Design review of the part built by this model. Coordinates are the model's own, in mm. A direction names the side the tool comes from. Give positions to 0.01 mm unless a question says otherwise; leave off trailing zeros. Order: outer loops, then holes, each group sorted by start corner. A loop starts at its lowest first (then second) coordinate and runs counter-clockwise, first axis right, second up. Notation, with made-up numbers: (22.5, 63) -> (36.5, 63) arc R29 ccw to (36.5, 99) -> close; hole circle Ø11 at (83.25, -6). An arc over 180 degrees is marked (long way). One line per item, written item: value.
from build123d import *

# Parameters (mm, degrees)
F0_R      = 3.175
F1_DEPTH  = 76.2
F2_R      = 3.175
F3_DEPTH  = 25.4
F3_FACE_R = 3.175
F4_DEPTH  = 50.8


with BuildPart() as f1:
    # F0 (on Front) → F1 (new body)
    with BuildSketch(Plane.XZ):
        Circle(F0_R)
    extrude(amount=F1_DEPTH)

    # F2 (on Right) → F3 (join)
    with BuildSketch(Plane.YZ):
        Circle(F2_R)
    extrude(amount=F3_DEPTH)

    # F3_face (on face) → F4 (join)
    with BuildSketch(Plane.YZ.offset(25.4)):
        Circle(F3_FACE_R)
    extrude(amount=F4_DEPTH)


solid = f1.part
Item 1: Clearance check with flat-ended pins moving along their axes: P1, Ø1.6, axis at x = -1.5, z = 1, coming from the +Y side; P2, Ø1.5, axis at x = 18.5, z = 1.5, coming from the -Y side; P3, Ø2.5, axis at y = 1.5, z = 0, coming from the -X side. State where each tip first meets the part, or that it passes through.
Returned:
P1: y = 0
P2: y = -3.09
P3: x = 0
Item 2: To check wall thickness, follow line 1 along X through (y, z) = (-34.5, 0) (3 decimals); line 2 along Y through (x, z) = (33, -2.75). State the ranges of each line that lie inside material, in increasing order. Write a range as from..to.
Returned:
line 1: -3.175..3.175
line 2: -1.59..1.59
Item 3: Add section B-B on y = -38. Give the boundary of the cut face in (x, z) (3 decimals).
Returned:
outline: circle Ø6.35 at (0, 0)
Item 4: Add section A-A on z = 0. Give the boundary of the cut face in (x, y) (3 decimals), plus the area to 3 significant figures.
Returned:
outline: (-3.175, -76.2) -> (3.175, -76.2) -> (3.175, -3.175) -> (76.2, -3.175) -> (76.2, 3.175) -> (0, 3.175) -> (0, 0) -> (-3.175, 0) -> close
area: 958 mm²
Item 5: Machinability: for faces 1 (the cylindrical face through (37.57, -0.69, -3.1)), 2 (the cylindrical face through (-0.69, -37.57, -3.1)), 3 (the flat face through (-1, 0, 0)), which of the approach directions +Z, -Z, +X, -X, +Y, -Y give a long, thin tool a straight path to every point of the face, cutting with its end or side? Answer none if there is none.
Returned:
face 1: +X
face 2: -Y
face 3: +Z, -Z, -X, +Y
